Could you check a few things on this model? Use its own coordinates, in mm. A direction names the side the tool comes from. Coordinates: 2 decimals unless noted, no trailing zeros. Order: outer loops, then holes, each group sorted by start corner. A loop starts at its lowest first (then second) coordinate and runs counter-clockwise, first axis right, second up. Notation, with made-up numbers: (85.25, -27) - (134.25, -27) arc R7 cw to (134.25, -23) - close; hole circle Ø8 at (-31.5, -5). An arc over 180 degrees is marked (long way). One line per item, written item: value. Start each with the question number.
Autodesk Inventor part; units mm, degrees
ref_plane "YZ Plane" through (0, 0, 0) normal (1, 0, 0) x (0, 1, 0)
ref_plane "XZ Plane" through (0, 0, 0) normal (0, 1, 0) x (-1, 0, 0)
ref_plane "XY Plane" through (0, 0, 0) normal (0, 0, 1) x (1, 0, 0)
sketch "Sketch1" plane through (0, 0, 0) normal (0, 1, 0) x (-1, 0, 0)
  line L0 (613.6799, 122.9576) -> (173.739, 376.9576)
  line L1 (-2.2373, 275.3576) -> (-2.2373, -232.6424)
  line L2 (173.739, -334.2424) -> (613.6799, -80.2424)
  line L3 (613.6799, 122.9576) -> (613.6799, -80.2424)
  line L4 (173.739, 376.9576) -> (-2.2373, 275.3576)
  line L5 (173.739, -334.2424) -> (-2.2373, -232.6424)
  line L6 (588.2799, 108.2929) -> (173.739, 347.6282)
  line L7 (173.739, 347.6282) -> (23.1627, 260.6929)
  line L8 (23.1627, 260.6929) -> (23.1627, -217.9777)
  line L9 (23.1627, -217.9777) -> (173.739, -304.913)
  line L10 (173.739, -304.913) -> (588.2799, -65.5777)
  line L11 (588.2799, -65.5777) -> (588.2799, 108.2929)
  line L12 (397.9021, 218.2076) -> (397.9021, -175.4924)
  line L13 (364.1169, 237.7135) -> (23.1627, 40.8635)
  line L14 (364.1169, -194.9983) -> (23.1627, 1.8517)
  line L15 (338.7169, 252.3782) -> (23.1627, 70.1929)
  line L16 (23.1627, -27.4777) -> (338.7169, -209.663)
  line L17 (423.3021, 203.5429) -> (423.3021, -160.8277)
  point P0 (0, 0)
  dimension "d0" = 203.2
  dimension "d6" = 508
  dimension "d14" = 393.7
  dimension "d16" = 393.7
  dimension "d17" = 393.7
extrude "Extrusion1" add sketch "Sketch1" along normal blind 50.8 contours L3 L2 L5 L1 L4 L0 | L17 L10 L12 L6 | L13 L8 L15 L6 | L10 L16 L8 L14
sketch "Sketch2" plane through (2.2373, 0, 275.3576) normal (0.5, 0, 0.866) x (0.866, 0, -0.5)
  line L0 (-203.2, 0) -> (0, 0)
  line L1 (0, 0) -> (0, 50.8)
  line L2 (-203.2, 50.8) -> (0, 50.8)
  line L3 (-203.2, 0) -> (-203.2, 50.8)
  line L4 (-203.2, 50.8) -> (0, 50.8)
  line L5 (-101.6, 50.8) -> (-101.6, 0)
  line L6 (-101.6, 25.4) -> (-152.4, 25.4)
  line L7 (-101.6, 25.4) -> (-50.8, 25.4)
  circle A0 centre (-50.8, 25.4) radius 12.7
  circle A1 centre (-152.4, 25.4) radius 12.7
  point P0 (135.7412, 0)
  dimension "d23" = 50.8
  dimension "d24" = 50.8
  dimension "d25" = 25.4
  dimension "d26" = 25.4
extrude "Extrusion2" cut sketch "Sketch2" against normal blind 25.4 contours A1 | A0
sketch "Sketch3" plane through (-173.739, 0, -334.2424) normal (0.5, 0, -0.866) x (-0.866, 0, -0.5)
  line L0 (-203.2, 0) -> (0, 0)
  line L1 (0, 0) -> (0, 50.8)
  line L2 (-203.2, 50.8) -> (0, 50.8)
  line L3 (-203.2, 0) -> (-203.2, 50.8)
  line L4 (152.4, 50.8) -> (-355.6, 50.8)
  line L5 (-101.6, 50.8) -> (-101.6, 0)
  line L6 (152.4, 0) -> (-355.6, 0)
  line L7 (-101.6, 25.4) -> (-152.4, 25.4)
  line L8 (-101.6, 25.4) -> (-50.8, 25.4)
  circle A0 centre (-50.8, 25.4) radius 12.7
  circle A1 centre (-152.4, 25.4) radius 12.7
  point P0 (-317.5836, 0)
  dimension "d29" = 50.8
  dimension "d30" = 50.8
  dimension "d31" = 25.4
  dimension "d32" = 25.4
extrude "Extrusion3" cut sketch "Sketch3" against normal blind 25.4 contours A1 | A0
sketch "Sketch4" plane through (-613.6799, 0, -80.2424) normal (-1, 0, 0) x (0, 0, 1)
  line L0 (150.4353, 0) -> (150.4353, 50.8)
  line L1 (0, 0) -> (203.2, 0)
  line L2 (203.2, 0) -> (203.2, 50.8)
  line L3 (0, 50.8) -> (203.2, 50.8)
  line L4 (0, 0) -> (0, 50.8)
  line L5 (355.6, 50.8) -> (-152.4, 50.8)
  line L6 (101.6, 50.8) -> (101.6, 0)
  line L7 (355.6, 0) -> (-152.4, 0)
  line L8 (101.6, 25.4) -> (50.8, 25.4)
  line L9 (101.6, 25.4) -> (152.4, 25.4)
  circle A0 centre (152.4, 25.4) radius 12.7
  circle A1 centre (50.8, 25.4) radius 12.7
  point P0 (80.2424, 0)
  dimension "d35" = 50.8
  dimension "d36" = 50.8
  dimension "d37" = 25.4
  dimension "d38" = 25.4
extrude "Extrusion4" cut sketch "Sketch4" against normal blind 25.4 contours A0 L9 L0 | L0 A0 | A1 | L9 A0 L0
properties part number "Top" material "Steel"
Q1. Which directions (+Z, -Z, +X, -X, +Y, -Y) give clear straight access to the entire face, cutting with the end or side of a thin tool? Please do faces 5 (the cylindrical face through (-37.527, 29.215, 283.856)), 6 (the flat face through (-23.163, 25, 22)).
Q2. I want a section at B-B on x = -204. Please give me the cut outline in (y, z), then the cut area to 3 significant figures.
Q3. We'd pull the mould along Y, two halves only. Please class faces 1 (the flat face through (-167, 0, 128)), 2 (the flat face through (-167, 50.8, 128)), 3 (the cylindrical face through (-601.16, 37.99, 70.5)), 4 (the cylindrical face through (-601.2, 36.1, -22.6)): +Y half, -Y half, draft (parallel to the pull), parting line (faces both ways), or undercut.
Q4. I want a section at C-C on y = 25.4. State how many separate pieces and enclosed holes the cut face has, then the cut area to 3 significant figures.
Q5. I want a section at A-A on x = -570. Please give me the cut outline in (y, z).
Q6. I'm going to push flat-ended pins straight in: pin 1 (23 mm diameter, centred on y = 25.4, z = -29.44, fed in from -X); pin 2 (2 mm diameter, centred on y = 33, z = 265, fed in from -X). Where does each tip first touch, or does it pass through?
Q7. If I drill on L1, parallel to X at y = 23, z = 18; L2, parallel to X at y = 3, z = -48; L3, parallel to X at y = 21, z = -194.5, over which ranges is the centre line in solid material (lowest first)?
Values follow:
1. face 5: none
1. face 6: +Y, -Y
2. outline: (0, -316.77) - (50.8, -316.77) - (50.8, -287.44) - (0, -287.44) - close; (0, -131.88) - (50.8, -131.88) - (50.8, -102.55) - (0, -102.55) - close; (0, 145.27) - (50.8, 145.27) - (50.8, 174.6) - (0, 174.6) - close; (0, 330.16) - (50.8, 330.16) - (50.8, 359.49) - (0, 359.49) - close
2. area: 5,960 mm^2
3. face 1: -Y half
3. face 2: +Y half
3. face 3: undercut
3. face 4: undercut
4. separate pieces: 4
4. enclosed holes: 1
4. area: 77,000 mm^2
5. outline: (0, -105.46) - (50.8, -105.46) - (50.8, -76.13) - (0, -76.13) - close; (0, 118.85) - (50.8, 118.85) - (50.8, 148.18) - (0, 148.18) - close
6. pin 1: stops at x = -423.3
6. pin 2: stops at x = -369.39
7. L1: x = -613.68 to -588.28, -423.3 to -397.9, -23.16 to 2.24
7. L2: x = -613.68 to -588.28, -423.3 to -397.9, -109.51 to -58.71, -23.16 to 2.24
7. L3: x = -415.78 to -364.98, -363.25 to -312.45, -23.16 to 2.24
